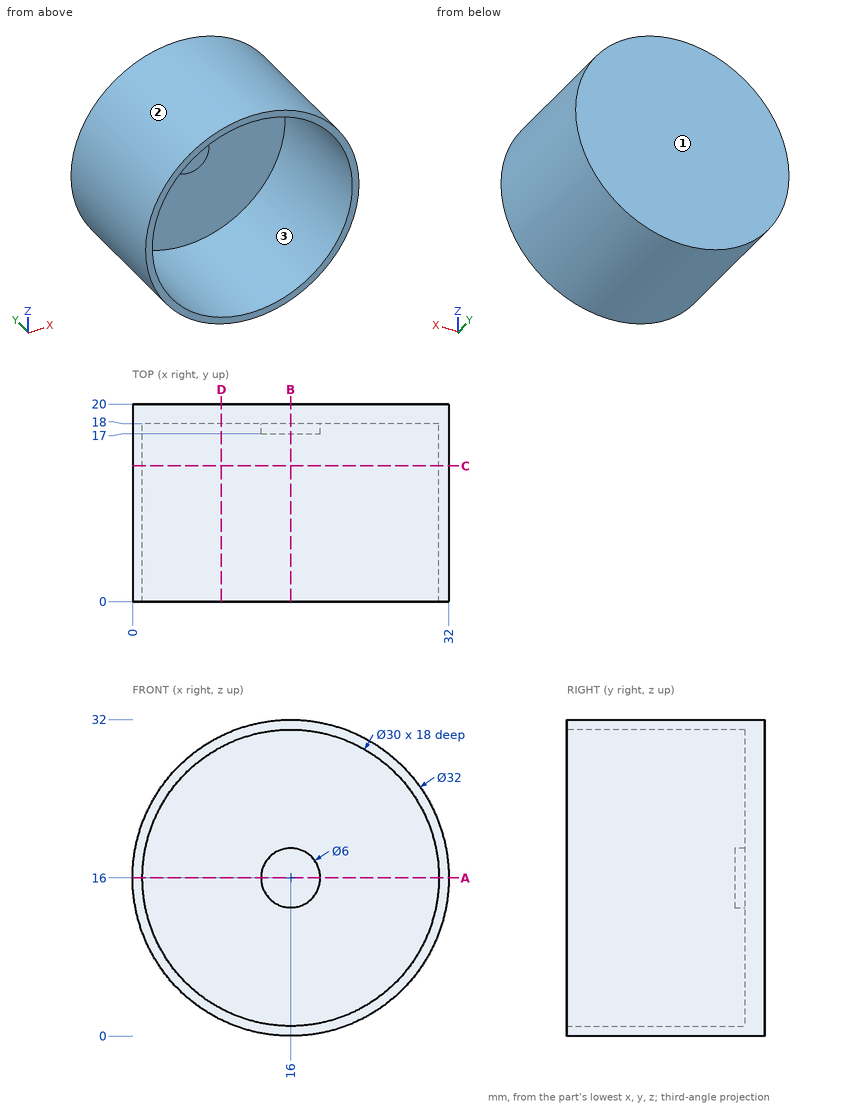
Verification items for this drawing (mm, ordinates from the low corner). Coordinates: 2 decimals unless noted, no trailing zeros. Loops run counter-clockwise (first coordinate to the right, second up) from the corner with the lowest first, then second, coordinate; pieces in that order, holes last. Notation, with made-up numbers: (31.25, -16) - (75.25, -16) arc R17 ccw to (75.25, 2) - close; hole circle Ø7 at (26.25, 58.25). An arc over 180 degrees is marked (long way). One line per item, written item: value. Start each with the question number.
(1) Cross-section at C-C on y = 13.75. Enter the section's corners in (x, z), plus the area to 3 significant figures.
(2) Material ranges on line 1 (X direction, y = 10.75, z = 16); line 2 (Y direction, x = 11, z = 11); line 3 (Z direction, x = 6, y = 5.5), recorded low to high. Write a range as [from, to].
(3) Depth check by flat-ended pin: P1, Ø6, axis at y = 14, z = 6.5, coming from the -X side; P2, Ø10, axis at x = 23, y = 2.5, coming from the -Z side; P3, Ø6, axis at x = 12, z = 7.5, coming from the -Y side; P4, Ø2, axis at x = 15, y = 3.5, coming from the -Z side. Enter the tip coordinate at first touch or a pass-through.
(4) Cross-section at D-D on x = 9. Enter the section's corners in (y, z).
(5) Mould release check, pull along X, two halves, no side actions. Record for the marked faces 1, 2 and 3: released by +X, released by -X, zero draft, split by the parting line, or undercut.
(6) Cross-section at A-A on z = 16. Enter the section's corners in (x, y), plus the area to 3 significant figures.
(7) Cross-section at B-B on x = 16. Enter the section's corners in (y, z).
Results below:
1. outline: circle Ø32 at (16, 16); hole circle Ø30 at (16, 16)
1. area: 97.4 mm2
2. line 1: x = [0, 1], [31, 32]
2. line 2: y = [18, 20]
2. line 3: z = [3.51, 4.82], [27.18, 28.49]
3. P1: stops at x = 1.38
3. P2: stops at z = 0.13
3. P3: stops at y = 18
3. P4: stops at z = 0
4. outline: (0, 1.61) - (20, 1.61) - (20, 30.39) - (0, 30.39) - (0, 29.27) - (18, 29.27) - (18, 2.73) - (0, 2.73) - close
5. face 1: zero draft
5. face 2: split by the parting line
5. face 3: undercut
6. outline: (0, 0) - (1, 0) - (1, 18) - (13, 18) - (13, 17) - (19, 17) - (19, 18) - (31, 18) - (31, 0) - (32, 0) - (32, 20) - (0, 20) - close
6. area: 106 mm2
7. outline: (0, 0) - (20, 0) - (20, 32) - (0, 32) - (0, 31) - (18, 31) - (18, 19) - (17, 19) - (17, 13) - (18, 13) - (18, 1) - (0, 1) - close
